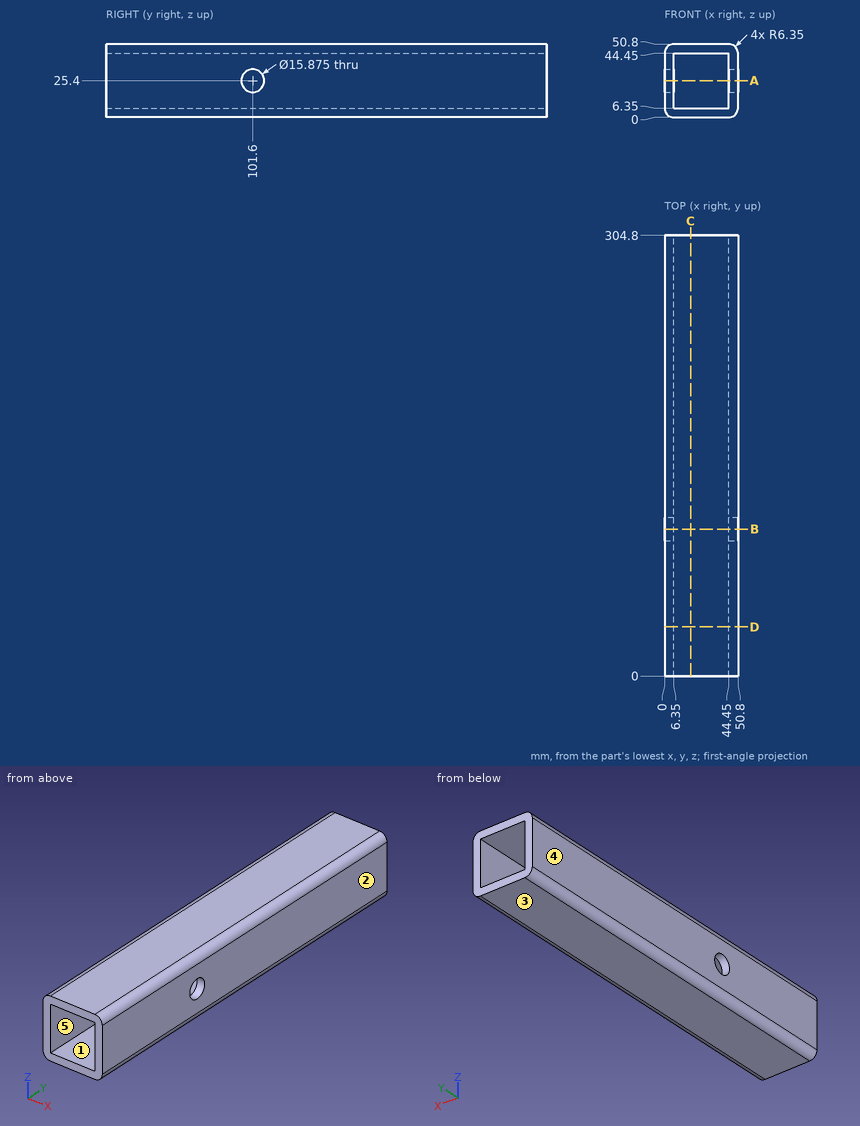
Source: three-view drawing plus pictorial views. Frame: mm from the lowest corner of the part. A direction names the side the tool comes from. Give positions to 0.01 mm unless a question says otherwise; leave off trailing zeros. Order: outer loops, then holes, each group sorted by start corner. A loop starts at its lowest first (then second) coordinate and runs counter-clockwise, first axis right, second up. Notation, with made-up numbers: M -2.75,-5 L 11.25,-5 A21 cw 11.25,17 Z; hole C 43,9.5 d6. An arc over 180 degrees is marked long. Return JSON: item names as keys, results as strings.
1) Section query C-C on x = 18. Output: boundary loops of the cut face in (y, z).
Taken from the geometry:
{"outline": "M 0,0 L 304.8,0 L 304.8,6.35 L 0,6.35 Z; M 0,44.45 L 304.8,44.45 L 304.8,50.8 L 0,50.8 Z"}
2) Line query: L1, parallel to X at y = 240.5, z = 7; L2, parallel to Y at x = 46, z = 25. Output: solid intervals per line, ascending. Write a range as [from, to].
Taken from the geometry:
{"L1": "x = [0, 6.35], [44.45, 50.8]", "L2": "y = [0, 93.67], [109.53, 304.8]"}
3) Section query D-D on y = 34. Output: boundary loops of the cut face in (x, z), and give its area (3 significant figures).
Taken from the geometry:
{"outline": "M 0,6.35 A6.35 ccw 6.35,0 L 44.45,0 A6.35 ccw 50.8,6.35 L 50.8,44.45 A6.35 ccw 44.45,50.8 L 6.35,50.8 A6.35 ccw 0,44.45 Z; hole M 6.35,6.35 L 44.45,6.35 L 44.45,44.45 L 6.35,44.45 Z", "area": "1,090 mm2"}
4) Section query A-A on z = 25.4. Output: boundary loops of the cut face in (x, y).
Taken from the geometry:
{"outline": "M 0,0 L 6.35,0 L 6.35,93.66 L 0,93.66 Z; M 0,109.54 L 6.35,109.54 L 6.35,304.8 L 0,304.8 Z; M 44.45,0 L 50.8,0 L 50.8,93.66 L 44.45,93.66 Z; M 44.45,109.54 L 50.8,109.54 L 50.8,304.8 L 44.45,304.8 Z"}
5) Section query B-B on y = 101.6. Output: boundary loops of the cut face in (x, z), and give its area (3 significant figures).
Taken from the geometry:
{"outline": "M 0,6.35 A6.35 ccw 6.35,0 L 44.45,0 A6.35 ccw 50.8,6.35 L 50.8,17.46 L 44.45,17.46 L 44.45,6.35 L 6.35,6.35 L 6.35,17.46 L 0,17.46 Z; M 0,33.34 L 6.35,33.34 L 6.35,44.45 L 44.45,44.45 L 44.45,33.34 L 50.8,33.34 L 50.8,44.45 A6.35 ccw 44.45,50.8 L 6.35,50.8 A6.35 ccw 0,44.45 Z", "area": "893 mm2"}
6) Mould query, pull axis Z, two halves, no side actions, for the marked faces 1, 2 and 3. Classes: released by +Z, released by -Z, zero draft, split by the parting line, or undercut.
Taken from the geometry:
{"face 1": "undercut", "face 2": "zero draft", "face 3": "released by -Z"}
7) Access query for the marked faces 4 and 5. Directions: +Z, -Z, +X, -X, +Y, -Y. A direction counts if a zero-diameter tool reaches every point of the face in a straight line with its end or side. Return the directions, or none.
Taken from the geometry:
{"face 4": "+Z, -Z, -X, +Y, -Y", "face 5": "+Y, -Y"}
